The listing builds one solid part. Answer for the finished solid, in the listing's coordinates (mm). Face numbers are marked on the shaded views. A direction names the side the tool comes from. Coordinates: 2 decimals unless noted, no trailing zeros. Order: outer loops, then holes, each group sorted by start corner. A loop starts at its lowest first (then second) coordinate and runs counter-clockwise, first axis right, second up.
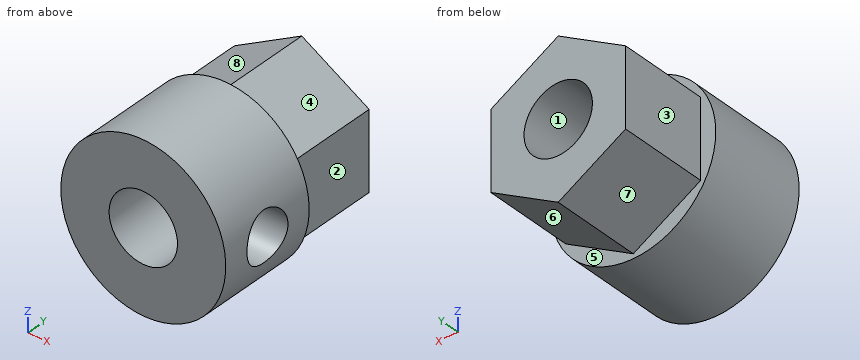
Solid Edge part; units mm, degrees
sketch "Sketch1" plane through (0, 0, 0) normal (0, -1, 0) x (1, 0, 0)
  line L0 (3.35, 1.9341) -> (0, 3.8682)
  line L1 (0, 3.8682) -> (-3.35, 1.9341)
  line L2 (-3.35, 1.9341) -> (-3.35, -1.9341)
  line L3 (-3.35, -1.9341) -> (0, -3.8682)
  line L4 (0, -3.8682) -> (3.35, -1.9341)
  line L5 (3.35, -1.9341) -> (3.35, 1.9341)
extrude "Protrusion1" add sketch "Sketch1" against normal blind 4.5
sketch "Sketch2" plane through (0, 0, 0) normal (0, -1, 0) x (0.866, 0, -0.5)
  circle A0 centre (0, 0) radius 4.1
extrude "ExtrudedProtrusion_3" add sketch "Sketch2" along normal blind 5
hole "Hole_1" at (0, -5, 0) direction (0, 1, 0) diameter 3.4 end up to next
hole "Hole_2" at (4.1, -2.5, 0) direction (-1, 0, 0) diameter 2.459 end up to next thread major 3 thread length 2
(1) Find section D-D (x = 2). Write down the section's boundary in (y, z), and give its area (3 significant figures).
(2) The mould has two halves that part along X. Classify the marked faces 1, 2 and 3: released by +X, released by -X, zero draft, split by the parting line, or undercut.
(3) Find section B-B (y = 2.25). Write down the section's boundary in (x, z), and give its area (3 significant figures).
(4) Each of these flat-tipped pins is pushed along its axis until it touches: pin 1 Ø1.2 at (y, z) = (3.5, 0) entering from -X; pin 2 Ø1.9 at (y, z) = (3, -1) entering from +X. Where does it stop, or does it pass through?
(5) For the marked faces 4, 5, 6, 7 and 8, determine the directions among +Z, -Z, +X, -X, +Y, -Y from which every point of the face is accessible in a straight line to the end or side of a thin tool.
(6) Find section A-A (z = 0). Write down the section's boundary in (x, y).
(7) Find section C-C (x = -1.25). Write down the section's boundary in (y, z).
(8) Consider line 1 (X direction, y = 2.75, z = 0); line 2 (Y direction, x = -1.5, z = -3.25); line 3 (X direction, y = 1.5, z = -1.5). Determine where each line is inside the solid, lowest interval first.
Findings below:
1. outline: (-5, -3.58) - (0, -3.58) - (0, -2.71) - (4.5, -2.71) - (4.5, 2.71) - (0, 2.71) - (0, 3.58) - (-5, 3.58) - close; hole circle Ø2.46 at (-2.5, 0)
1. area: 55.5 mm2
2. face 1: undercut
2. face 2: released by +X
2. face 3: released by -X
3. outline: (-3.35, -1.93) - (0, -3.87) - (3.35, -1.93) - (3.35, 1.93) - (0, 3.87) - (-3.35, 1.93) - close; hole circle Ø3.4 at (0, 0)
3. area: 29.8 mm2
4. pin 1: stops at x = -3.35
4. pin 2: stops at x = 3.35
5. face 4: +Z, +X, +Y
5. face 5: +Y
5. face 6: -Z, +X, +Y
5. face 7: -Z, -X, +Y
5. face 8: +Z, -X, +Y
6. outline: (-4.1, -5) - (-1.7, -5) - (-1.7, 4.5) - (-3.35, 4.5) - (-3.35, 0) - (-4.1, 0) - close; (1.7, -5) - (4.1, -5) - (4.1, -3.73) - (1.7, -3.73) - close; (1.7, -1.27) - (4.1, -1.27) - (4.1, 0) - (3.35, 0) - (3.35, 4.5) - (1.7, 4.5) - close
7. outline: (-5, -3.9) - (0, -3.9) - (0, -3.15) - (4.5, -3.15) - (4.5, -1.15) - (-5, -1.15) - close; (-5, 1.15) - (4.5, 1.15) - (4.5, 3.15) - (0, 3.15) - (0, 3.9) - (-5, 3.9) - close
8. line 1: x = -3.35 to -1.7, 1.7 to 3.35
8. line 2: y = -5 to 0
8. line 3: x = -3.35 to -0.8, 0.8 to 3.35
